CAD build for the part. Positions are in the model's coordinates, mm. A direction names the side the tool comes from. Round coordinates to 2 decimals unless told otherwise and drop trailing zeros. Loops run counter-clockwise (first coordinate to the right, second up) from the corner with the lowest first, then second, coordinate; pieces in that order, holes last. Notation, with made-up numbers: M 52,54 L 82,54 A10 cw 82,61 Z; hole C 56.25,56.5 d6. An arc over 180 degrees is marked long. Put each result on its own line as item: value. Start each with the question number.
from build123d import *

# Parameters (mm, degrees)
F1_DEPTH = 6.35
F3_DEPTH = 6.35
F4_R     = 3.175


with BuildPart() as f1:
    # F0 (on Front) → F1 (new body)
    with BuildSketch(Plane.XZ):
        with BuildLine():
            Line((0, 88.9), (0, 0))
            Line((0, 0), (152.4, 0))
            Line((152.4, 0), (152.4, 88.9))
            ThreePointArc((152.4, 88.9), (148.680256, 97.880256), (139.7, 101.6))
            Line((139.7, 101.6), (12.7, 101.6))
            ThreePointArc((12.7, 101.6), (3.719744, 97.880256), (0, 88.9))
        make_face()
        with BuildLine():
            ThreePointArc((15.875, 78.277995), (19.680409, 82.547098), (23.800897, 78.58125))
            Line((23.800897, 78.58125), (23.800897, 22.784778))
            ThreePointArc((23.800897, 22.784778), (19.721844, 19.051731), (15.8703, 23.019088))
            Line((15.8703, 23.019088), (15.875, 78.277995))
        make_face(mode=Mode.SUBTRACT)
        with BuildLine():
            Line((128.599103, 22.784778), (128.599103, 78.58125))
            ThreePointArc((128.599103, 78.58125), (132.719591, 82.547098), (136.525, 78.277995))
            Line((136.525, 78.277995), (136.5297, 23.019088))
            ThreePointArc((136.5297, 23.019088), (132.678156, 19.051731), (128.599103, 22.784778))
        make_face(mode=Mode.SUBTRACT)
    extrude(amount=F1_DEPTH)

    # F2 (on face) → F3 (join)
    with BuildSketch(Plane(origin=(0, 0, 0), x_dir=(1, 0, 0), z_dir=(0, 0, -1))):
        with BuildLine():
            Line((0, 0), (152.4, 0))
            Line((152.4, 0), (152.4, 25.4))
            ThreePointArc((152.4, 25.4), (76.2, 101.6), (0, 25.4))
            Line((0, 25.4), (0, 0))
        make_face()
    extrude(amount=-F3_DEPTH)

    # F4
    f4_edges = [f1.edges().sort_by_distance(p)[0] for p in [
        (76.2, 0, 0),
        (76.2, -6.35, 6.35),
    ]]
    fillet(f4_edges, radius=F4_R)


solid = f1.part
(1) Cut at D-D on y = -13. List the corners of the cut face in (x, z).
(2) Cut at A-A on z = 74. List the corners of the cut face in (x, y), and give its area (3 significant figures).
(3) Cut at B-B on x = 76.2. List the corners of the cut face in (y, z) (3 decimals).
(4) Flat gauge pins, fed straight in: pin 1 Ø8 at (x, z) = (46.5, 83) entering from -Y; pin 2 Ø1 at (x, y) = (113.5, -88.5) entering from +Z. Where does each tip first touch, or does it go through?
(5) Mould opens along Z. For faces 4 (the cylindrical face through (77.27, -7.3, 7.26)), 5 (the flat face through (23.801, -3, 51)), 6 (the flat face through (128.599, -3, 50)), 7 (the flat face through (152.4, -5, 38)) say: +Z half, -Z half, draft (parallel to the pull), parting line (faces both ways), or undercut.
(6) Drill centre lines: line 1 along Y through (x, z) = (24, 9.5); line 2 along Z through (x, y) = (29, -18.5). Where is each one in solid material? Low to high.
(7) Tool access for faces 1 (the flat face through (77, -3, 101.6)), 2 (the cylindrical face through (132.764, -3.131, 19.055)), 3 (the flat face through (75, -46, 6.35)): list every direction of +Z, -Z, +X, -X, +Y, -Y with a clear straight run to the whole face (end or side of a thin tool).
(8) Cut at C-C on x = 18. List the corners of the cut face in (y, z) (3 decimals).
Taken from the geometry:
1. outline: M 0,0 L 152.4,0 L 152.4,6.35 L 0,6.35 Z
2. outline: M 0,-6.35 L 15.87,-6.35 L 15.87,0 L 0,0 Z; M 23.8,-6.35 L 128.6,-6.35 L 128.6,0 L 23.8,0 Z; M 136.53,-6.35 L 152.4,-6.35 L 152.4,0 L 136.53,0 Z
2. area: 867 mm2
3. outline: M -101.6,0 L -3.175,0 A3.175 ccw 0,3.175 L 0,101.6 L -6.35,101.6 L -6.35,9.525 A3.175 cw -9.525,6.35 L -101.6,6.35 Z
4. pin 1: y = -6.35
4. pin 2: z = 6.35
5. face 4: +Z half
5. face 5: undercut
5. face 6: undercut
5. face 7: draft
6. line 1: -6.35 to 0
6. line 2: 0 to 6.35
7. face 1: +Z, +X, -X, +Y, -Y
7. face 2: +Y, -Y
7. face 3: +Z, +X, -X, -Y
8. outline: M -74.585,0 L -3.175,0 A3.175 ccw 0,3.175 L 0,19.502 L -6.35,19.502 L -6.35,9.525 A3.175 cw -9.525,6.35 L -74.585,6.35 Z; M -6.35,82.102 L 0,82.102 L 0,101.6 L -6.35,101.6 Z
